Here's how the part is built. I have some questions about the finished solid (model axes, mm). Face numbers are marked on the shaded views. Give positions to 0.01 mm unless a question says otherwise; leave off trailing zeros. Write each loop counter-clockwise with the first axis right and the second up, starting at its lowest first coordinate (ties: lowest second). Pieces come first, ordered by that corner, then holes. Notation, with made-up numbers: (17, 77) -> (43, 77) arc R14 ccw to (43, 92) -> close; hole circle Ø2 at (39, -23.75). An arc over 180 degrees is marked (long way). Use CSV: the item, a comma, the result in double quotes. Start each with the question number.
(1) For pin 1 Ø1.5 at (x, z) = (8.5, 1.5) entering from +Y; pin 2 Ø1.5 at (x, y) = (7.5, -4) entering from +Z; pin 3 Ø3 at (x, y) = (0.5, 4.5) entering from -Z, each with a flat end and sliding along its axis, tell me the tip position at first contact or that it passes through.
(2) Suppose I cut it at C-C on x = 5.5. List the corners of the cut face in (y, z) for me, plus the area to 3 significant figures.
(3) I need wall thicknesses on L1, parallel to Z at x = -0.55, y = 0; L2, parallel to Z at x = 4.25, y = 0; L3, parallel to X at y = 9.25, z = -2.75. Which ranges of each line are inside material? Lowest first, please. Write a range as [from, to].
(4) If we mould it in two halves opening along Z, with no side actions, what happens to the marked faces 1, 2 and 3? For each: pulls with the +Z half, pulls with the -Z half, needs draft (parallel to the pull), parting line crosses it, or undercut.
(5) Suppose I cut it at D-D on z = -10. List the corners of the cut face in (x, y) for me, plus the area to 3 significant figures.
(6) Suppose I cut it at A-A on y = 0. List the corners of the cut face in (x, z) for me.
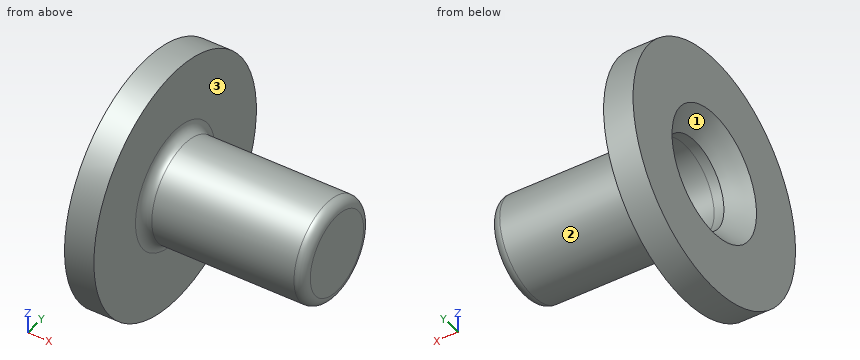
from build123d import *

# Parameters (mm, degrees)
F0_R     = 5.1
F0_R_2   = 4.5
F1_DEPTH = 15
F2_R     = 5.1
F3_DEPTH = 1.5
F4_R     = 12.5
F4_R_2   = 4.5
F5_DEPTH = 3
F6_R     = 1
F7_SIZE  = 2


with BuildPart() as f1:
    # F0 (on Right) → F1 (new body)
    with BuildSketch(Plane.YZ):
        Circle(F0_R)
        Circle(F0_R_2, mode=Mode.SUBTRACT)
    extrude(amount=F1_DEPTH)

    # F2 (on face) → F3 (join)
    with BuildSketch(Plane.YZ.offset(15)):
        Circle(F2_R)
    extrude(amount=F3_DEPTH)

    # F4 (on face) → F5 (join)
    with BuildSketch(Plane(origin=(0, 0, 0), x_dir=(0, -1, 0), z_dir=(-1, 0, 0))):
        Circle(F4_R)
        Circle(F4_R_2, mode=Mode.SUBTRACT)
    extrude(amount=F5_DEPTH)

    # F6
    f6_edges = [f1.edges().sort_by_distance(p)[0] for p in [
        (16.5, -5.1, 0),
        (0, -5.1, 0),
    ]]
    fillet(f6_edges, radius=F6_R)

    # F7
    f7_edges = [f1.edges().sort_by_distance(p)[0] for p in [
        (-3, 4.5, 0),
    ]]
    chamfer(f7_edges, length=F7_SIZE)


solid = f1.part
Geometry says:
1,pin 1,"y = 5.04"
1,pin 2,"z = 3.93"
1,pin 3,"z = -12.11"
2,outline,"circle Ø10.2 at (0, 0); hole circle Ø9 at (0, 0)"
2,area,"18.1 mm²"
3,L1,"[-12.5, -4.5], [4.5, 12.5]"
3,L2,"[-5.1, -4.5], [4.5, 5.1]"
3,L3,"[-3, 0]"
4,face 1,"undercut"
4,face 2,"parting line crosses it"
4,face 3,"needs draft"
5,outline,"(-3, -7.5) -> (0, -7.5) -> (0, 7.5) -> (-3, 7.5) -> close"
5,area,"45.0 mm²"
6,outline,"(-3, -12.5) -> (0, -12.5) -> (0, -6.1) arc R1 cw to (1, -5.1) -> (15.5, -5.1) arc R1 ccw to (16.5, -4.1) -> (16.5, 4.1) arc R1 ccw to (15.5, 5.1) -> (1, 5.1) arc R1 cw to (0, 6.1) -> (0, 12.5) -> (-3, 12.5) -> (-3, 6.5) -> (-1, 4.5) -> (15, 4.5) -> (15, -4.5) -> (-1, -4.5) -> (-3, -6.5) -> close"
